from build123d import *

# Parameters (mm, degrees)
SKETCH_1_W      = 30
SKETCH_1_H      = 30
SKETCH_1_R      = 1.6
EXTRUDE_1_DEPTH = 2
FILLET_1_SIZE   = 3


with BuildPart() as part:
    # 草图1 → 凸台-拉伸1 (new body)
    with BuildSketch(Plane.XY):
        Rectangle(SKETCH_1_W, SKETCH_1_H)
        with Locations((-11.899958033, 11.899958033)):
            Circle(SKETCH_1_R, mode=Mode.SUBTRACT)
        with Locations(Location((11.899958033, 11.899958033, 0), (0, 0, 180))):
            Circle(SKETCH_1_R, mode=Mode.SUBTRACT)
        with Locations((11.899958033, -11.899958033)):
            Circle(SKETCH_1_R, mode=Mode.SUBTRACT)
        with Locations(Location((-11.899958033, -11.899958033, 0), (0, 0, 180))):
            Circle(SKETCH_1_R, mode=Mode.SUBTRACT)
    extrude(amount=EXTRUDE_1_DEPTH)

    # 圆角1
    # a fillet whose section is not a circle: 3 mm, written as the material it takes off along each edge
    with BuildSketch(Plane(origin=(-15, -15, -7.5), x_dir=(1, 0, 0), z_dir=(0, 0, 1)), Plane(origin=(15, -15, -7.5), x_dir=(0, 1, 0), z_dir=(0, 0, 1)), Plane(origin=(15, 15, -7.5), x_dir=(-1, 0, 0), z_dir=(0, 0, 1))) as fillet_1_piece_1:
        with BuildLine():
            Bezier((FILLET_1_SIZE, 0), (0, 0), (0, FILLET_1_SIZE), weights=[1, 0.818181818, 1])
            Line((0, FILLET_1_SIZE), (0, 0))
            Line((0, 0), (FILLET_1_SIZE, 0))
        make_face()
    extrude(amount=17, mode=Mode.SUBTRACT)
    with BuildSketch(Plane(origin=(-15, 15, -7.5), x_dir=(1, 0, 0), z_dir=(0, 0, 1))) as fillet_1_piece_2:
        with BuildLine():
            Bezier((FILLET_1_SIZE, 0), (0, 0), (0, -FILLET_1_SIZE), weights=[1, 0.818181818, 1])
            Line((0, -FILLET_1_SIZE), (0, 0))
            Line((0, 0), (FILLET_1_SIZE, 0))
        make_face()
    extrude(amount=17, mode=Mode.SUBTRACT)


solid = part.part
Input: part model. Units: mm. Frame: model coordinates. Give positions to 0.01 mm unless a question says otherwise; leave off trailing zeros.
Q1. Material intervals for probe 1 along X at (y, z) = (13, 0.6); probe 2 along Y at (x, z) = (11, 1.7); probe 3 along Y at (x, z) = (-11.5, 0.9), sorted ascending.
Q2. Pull-direction query (Y, two-part tool) for faces 1 (the face through (0, -15, 1)), 2 (the face through (0, 0, 0)), 3 (the face through (12.64, -13.32, 0.99)), 4 (the face through (0, 15, 1)); classes: pulls with the +Y half, pulls with the -Y half, needs draft (parallel to the pull), parting line crosses it, or undercut.
Q3. Section A-A, the plane z = 0.75. State how many separate pieces and enclosed holes the cut face has, plus the area to 3 significant figures.
Filled in:
1. probe 1: x = -14.86 to -13.06, -10.74 to 10.74, 13.06 to 14.86
1. probe 2: y = -15 to -13.22, -10.58 to 10.58, 13.22 to 15
1. probe 3: y = -15 to -13.45, -10.35 to 10.35, 13.45 to 15
2. face 1: pulls with the -Y half
2. face 2: needs draft
2. face 3: undercut
2. face 4: pulls with the +Y half
3. separate pieces: 1
3. enclosed holes: 4
3. area: 861 mm2
